from build123d import *

# Parameters (mm, degrees)
BOSS_EXTRUDE1_DEPTH = 5.5
SKETCH2_R           = 20
BOSS_EXTRUDE2_DEPTH = 2.5
CUT_EXTRUDE1_DEPTH  = 8


with BuildPart() as part:
    # Sketch1 → Boss-Extrude1 (new body)
    with BuildSketch(Plane(origin=(0, 0, 0), x_dir=(1, 0, 0), z_dir=(0, 1, 0))):
        with BuildLine():
            ThreePointArc((-1.9, -2.05669638), (-2.8, 0), (-1.9, 2.05669638))
            Line((-1.9, 2.05669638), (-1.9, 5.532856405))
            ThreePointArc((-1.9, 5.532856405), (-5.85, 0), (-1.9, -5.532856405))
            Line((-1.9, -5.532856405), (-1.9, -2.05669638))
        make_face()
        with BuildLine():
            ThreePointArc((-1.9, 2.05669638), (0, 2.8), (1.9, 2.05669638))
            Line((1.9, 2.05669638), (1.9, 5.532856405))
            ThreePointArc((1.9, 5.532856405), (0, 5.85), (-1.9, 5.532856405))
            Line((-1.9, 5.532856405), (-1.9, 2.05669638))
        make_face()
        with BuildLine():
            Line((1.9, 5.532856405), (1.9, 2.05669638))
            ThreePointArc((1.9, 2.05669638), (2.565151068, 1.122497216), (2.8, 0))
            ThreePointArc((2.8, 0), (2.565151068, -1.122497216), (1.9, -2.05669638))
            Line((1.9, -2.05669638), (1.9, -5.532856405))
            ThreePointArc((1.9, -5.532856405), (4.761171074, -3.399080758), (5.85, 0))
            ThreePointArc((5.85, 0), (4.761171074, 3.399080758), (1.9, 5.532856405))
        make_face()
        with BuildLine():
            Line((1.9, -5.532856405), (1.9, -2.05669638))
            ThreePointArc((1.9, -2.05669638), (0, -2.8), (-1.9, -2.05669638))
            Line((-1.9, -2.05669638), (-1.9, -5.532856405))
            ThreePointArc((-1.9, -5.532856405), (0, -5.85), (1.9, -5.532856405))
        make_face()
        with BuildLine():
            Line((-1.9, -2.05669638), (-1.9, 2.05669638))
            ThreePointArc((-1.9, 2.05669638), (-2.8, 0), (-1.9, -2.05669638))
        make_face()
        with BuildLine():
            ThreePointArc((2.8, 0), (2.565151068, 1.122497216), (1.9, 2.05669638))
            Line((1.9, 2.05669638), (1.9, -2.05669638))
            ThreePointArc((1.9, -2.05669638), (2.565151068, -1.122497216), (2.8, 0))
        make_face()
    extrude(amount=BOSS_EXTRUDE1_DEPTH)

    # Sketch2 → Boss-Extrude2 (add)
    with BuildSketch(Plane(origin=(0, 5.5, 0), x_dir=(1, 0, 0), z_dir=(0, 1, 0))):
        with Locations(Location((0, 0, 0), (0, 0, 270))):
            Circle(SKETCH2_R)
    extrude(amount=-BOSS_EXTRUDE2_DEPTH)

    # Sketch3 → Cut-Extrude1 (cut)
    with BuildSketch(Plane.XZ.offset(-3)):
        with BuildLine():
            Line((-1.9, 2.05669638), (-1.9, -2.05669638))
            ThreePointArc((-1.9, -2.05669638), (0, -2.8), (1.9, -2.05669638))
            Line((1.9, -2.05669638), (1.9, 2.05669638))
            ThreePointArc((1.9, 2.05669638), (0, 2.8), (-1.9, 2.05669638))
        make_face()
    extrude(amount=-CUT_EXTRUDE1_DEPTH, mode=Mode.SUBTRACT)


solid = part.part
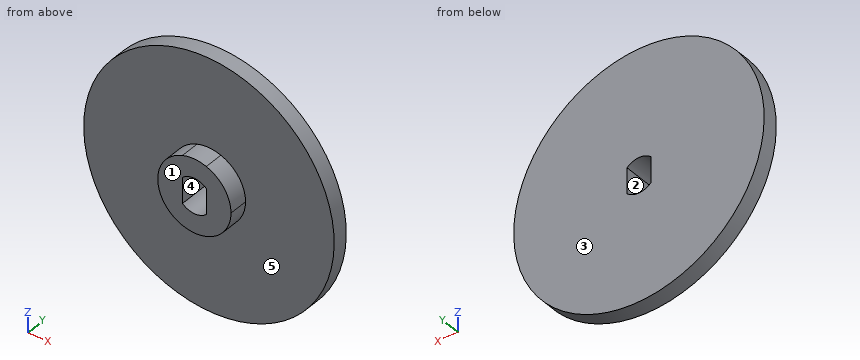
Can you work these out from the model? Positions are in its coordinate system, mm. Face numbers are marked on the shaded views. A direction names the side the tool comes from. Round coordinates to 2 decimals unless told otherwise and drop trailing zeros. Loops run counter-clockwise (first coordinate to the right, second up) from the corner with the lowest first, then second, coordinate; pieces in that order, holes last. Notation, with made-up numbers: (52, 59) - (82, 59) arc R21 cw to (82, 96) - close; hole circle Ø3 at (-13.5, 21). An arc over 180 degrees is marked (long way). Answer in a Markdown table with one row per item. Add a question column.
Q1. I want a section at A-A on x = 0. List the corners of the cut face in (y, z) for me.
Q2. I need wall thicknesses on L1, parallel to Y at x = 16, z = -2; L2, parallel to Z at x = -1.5, y = 3.75; L3, parallel to X at y = 5.35, z = 7 (3 decimals). Which ranges of each line are inside material? Lowest first, please.
Q3. We'd pull the mould along Z, two halves only. Please class the marked faces 1 and 2: pulls with the +Z half, pulls with the -Z half, needs draft (parallel to the pull), parting line crosses it, or undercut.
Q4. For pin 1 Ø3 at (x, y) = (-3.5, 3.5) entering from -Z; pin 2 Ø3 at (x, z) = (14.5, -5.5) entering from -Y, each with a flat end and sliding along its axis, tell me the tip position at first contact or that it passes through.
Q5. I want a section at B-B on y = 2.5. List the corners of the cut face in (x, z) for me, and give its area (3 significant figures).
Q6. I want a section at C-C on z = -16. List the corners of the cut face in (x, y) for me.
Q7. Which directions (+Z, -Z, +X, -X, +Y, -Y) give clear straight access to the entire face, cutting with the end or side of a thin tool? Please do the marked faces 3, 4 and 5.
Q8. I want a section at D-D on y = 4.8. List the corners of the cut face in (x, z) for me.
A:
| question | item | result |
|---|---|---|
| 1 | outline | (0, -5.85) - (3, -5.85) - (3, -20) - (5.5, -20) - (5.5, -2.8) - (0, -2.8) - close; (0, 2.8) - (5.5, 2.8) - (5.5, 20) - (3, 20) - (3, 5.85) - (0, 5.85) - close |
| 2 | L1 | 3 to 5.5 |
| 2 | L2 | -19.94 to -2.36, 2.36 to 19.94 |
| 2 | L3 | -18.735 to 18.735 |
| 3 | face 1 | needs draft |
| 3 | face 2 | undercut |
| 4 | pin 1 | z = -19.9 |
| 4 | pin 2 | y = 3 |
| 5 | outline | circle Ø11.7 at (0, 0); hole (-1.9, -2.06) arc R2.8 ccw to (1.9, -2.06) - (1.9, 2.06) arc R2.8 ccw to (-1.9, 2.06) - close |
| 5 | area | 88.0 mm^2 |
| 6 | outline | (-12, 3) - (12, 3) - (12, 5.5) - (-12, 5.5) - close |
| 7 | face 3 | +Z, -Z, +X, -X, +Y |
| 7 | face 4 | +Y, -Y |
| 7 | face 5 | -Y |
| 8 | outline | circle Ø40 at (0, 0); hole (-1.9, -2.06) arc R2.8 ccw to (1.9, -2.06) - (1.9, 2.06) arc R2.8 ccw to (-1.9, 2.06) - close |
